Geometry: final body of the model. Coordinates: model frame, mm. Face numbers are marked on the shaded views. Coordinates: 2 decimals unless noted, no trailing zeros. Loops run counter-clockwise (first coordinate to the right, second up) from the corner with the lowest first, then second, coordinate; pieces in that order, holes last. Notation, with made-up numbers: M 61.25,75 L 103.25,75 A21 ccw 103.25,105 Z; hole C 81,83.5 d1. An arc over 180 degrees is marked long. Write each question's results on one line, items separated by ' | '. Start each with the question number.
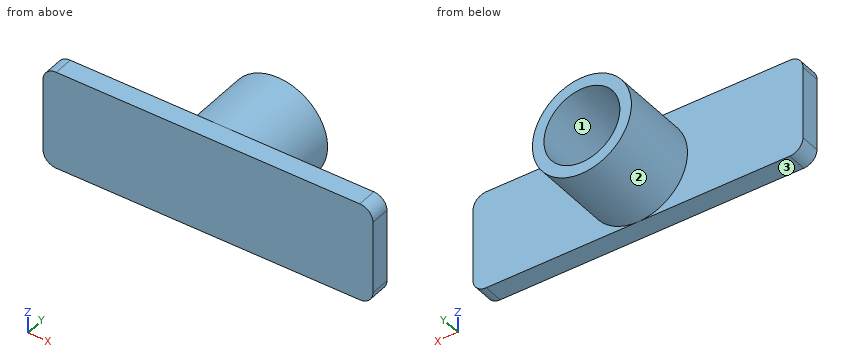
from build123d import *

# Parameters (mm, degrees)
SKIZZE1_W                       = 50
SKIZZE1_H                       = 15
AUFSATZ_LINEAR_AUSTRAGEN1_DEPTH = 3
SKIZZE2_R                       = 7.5
SKIZZE2_R_2                     = 5.75
AUFSATZ_LINEAR_AUSTRAGEN2_DEPTH = 12
VERRUNDUNG1_R                   = 2


with BuildPart() as part:
    # Skizze1 → Aufsatz-Linear austragen1 (new body)
    with BuildSketch(Plane(origin=(0, 0, 0), x_dir=(1, 0, 0), z_dir=(0, 1, 0))):
        Rectangle(SKIZZE1_W, SKIZZE1_H)
    extrude(amount=AUFSATZ_LINEAR_AUSTRAGEN1_DEPTH)

    # Skizze2 → Aufsatz-Linear austragen2 (add)
    with BuildSketch(Plane(origin=(0, 3, 0), x_dir=(1, 0, 0), z_dir=(0, 1, 0))):
        Circle(SKIZZE2_R)
        Circle(SKIZZE2_R_2, mode=Mode.SUBTRACT)
    extrude(amount=AUFSATZ_LINEAR_AUSTRAGEN2_DEPTH)

    # Verrundung1
    verrundung1_edges = [part.edges().sort_by_distance(p)[0] for p in [
        (25, 1.5, 7.5),
        (-25, 1.5, 7.5),
        (-25, 1.5, -7.5),
        (25, 1.5, -7.5),
    ]]
    fillet(verrundung1_edges, radius=VERRUNDUNG1_R)


solid = part.part
Item 1: Contact query for flat-ended pins moving along their axis: P1, Ø3.5, axis at x = 0, z = -2, coming from the +Y side; P2, Ø6, axis at x = -6.5, y = 8.5, coming from the -Z side; P3, Ø2, axis at y = 5, z = -4.5, coming from the -X side. Output: stop coordinate, or through.
Item 2: Section A-A, the plane y = 13. Return loops of the section in (x, z).
Item 3: Section C-C, the plane z = 0. Return loops of the section in (x, y), plus the area to 3 significant figures.
Item 4: Pull-direction query (Z, two-part tool) for the marked faces 1, 2 and 3; classes: released by +Z, released by -Z, zero draft, split by the parting line, or undercut.
Item 5: Section D-D, the plane x = 16. Return loops of the section in (y, z), plus the area to 3 significant figures.
Item 6: Section B-B, the plane x = 3. Return loops of the section in (y, z), plus the area to 3 significant figures.
Item 7: Ray query, L1, parallel to Z at x = 0, y = 12; L2, parallel to Y at x = -15, z = -7. Return the intervals inside material, ascending. Write a range as [from, to].
Solutions:
1) P1: stops at y = 3 | P2: stops at z = -6.63 | P3: stops at x = -6.63
2) outline: C 0,0 d15; hole C 0,0 d11.5
3) outline: M -25,0 L 25,0 L 25,3 L 7.5,3 L 7.5,15 L 5.75,15 L 5.75,3 L -5.75,3 L -5.75,15 L -7.5,15 L -7.5,3 L -25,3 Z | area: 192 mm²
4) face 1: undercut | face 2: split by the parting line | face 3: released by -Z
5) outline: M 0,-7.5 L 3,-7.5 L 3,7.5 L 0,7.5 Z | area: 45.0 mm²
6) outline: M 0,-7.5 L 3,-7.5 L 3,-6.87 L 15,-6.87 L 15,-4.91 L 3,-4.91 L 3,4.91 L 15,4.91 L 15,6.87 L 3,6.87 L 3,7.5 L 0,7.5 Z | area: 92.2 mm²
7) L1: z = [-7.5, -5.75], [5.75, 7.5] | L2: y = [0, 3]
